Work out the finished part from the listing and answer in its coordinate system (mm). A direction names the side the tool comes from. Coordinates: 2 decimals unless noted, no trailing zeros. Order: outer loops, then holes, each group sorted by start corner. A loop starts at its lowest first (then second) coordinate and runs counter-clockwise, first axis right, second up. Notation, with made-up numbers: M 13.25,14.5 L 66.25,14.5 A28 ccw 66.25,51.5 Z; hole C -23.5,52.25 d3. An arc over 180 degrees is marked long. Use a Markdown table: item, result. Add a question column.
from build123d import *

# Parameters (mm, degrees)
F0_W      = 8
F0_H      = 25
F1_DEPTH  = 1
F2_R      = 6.5
F2_R_2    = 4.3
F3_DEPTH  = 11
F4_R      = 4
F5_R      = 1.35
F6_DEPTH  = 50.001
F7_R      = 2
F8_W      = 1.5
F8_H      = 6
F9_DEPTH  = 2
F11_DEPTH = 2


with BuildPart() as f1:
    # F0 (on Top) → F1 (new body)
    with BuildSketch(Plane.XY):
        with Locations((-4, -12.5)):
            Rectangle(F0_W, F0_H)
        Polygon((-8, 0), (0, 0), (0, 13), (-8, 13), (-42, 13), (-50, 13), (-50, 0), (-42, 0), align=None)
        with Locations((-4, 25.5)):
            Rectangle(F0_W, F0_H)
        with Locations((-46, -12.5)):
            Rectangle(F0_W, F0_H)
        with Locations((-46, 25.5)):
            Rectangle(F0_W, F0_H)
    extrude(amount=F1_DEPTH)

    # F2 (on face) → F3 (join)
    with BuildSketch(Plane.XY.offset(1)):
        with Locations((-34.25, 6.5)):
            Circle(F2_R)
        with Locations((-34.25, 6.5)):
            Circle(F2_R_2, mode=Mode.SUBTRACT)
        with Locations((-15.75, 6.5)):
            Circle(F2_R)
        with Locations((-15.75, 6.5)):
            Circle(F2_R_2, mode=Mode.SUBTRACT)
    extrude(amount=F3_DEPTH)

    # F4
    f4_edges = [f1.edges().sort_by_distance(p)[0] for p in [
        (-38.55, 6.5, 1),
        (-20.05, 6.5, 1),
    ]]
    fillet(f4_edges, radius=F4_R)

    # F5 (on face) → F6 (cut, through all)
    with BuildSketch(Plane.YZ):
        with Locations((6.5, 8.15)):
            Circle(F5_R)
    extrude(amount=-F6_DEPTH, mode=Mode.SUBTRACT)

    # F7
    f7_edges = [f1.edges().sort_by_distance(p)[0] for p in [
        (-42, 38, 0.5),
        (0, 38, 0.5),
        (-8, 38, 0.5),
        (-42, 13, 0.5),
        (-8, 13, 0.5),
        (-8, 0, 0.5),
        (0, -25, 0.5),
        (-8, -25, 0.5),
        (-42, 0, 0.5),
        (-42, -25, 0.5),
        (-50, -25, 0.5),
        (-50, 38, 0.5),
    ]]
    fillet(f7_edges, radius=F7_R)

    # F8 (on face) → F9 (join)
    with BuildSketch(Plane.XY.offset(1)):
        with Locations((-49.25, 33)):
            Rectangle(F8_W, F8_H)
        with Locations((-42.75, 33)):
            Rectangle(F8_W, F8_H)
        with Locations((-42.75, -20)):
            Rectangle(F8_W, F8_H)
        with Locations((-49.25, -20)):
            Rectangle(F8_W, F8_H)
        with Locations((-0.75, 33)):
            Rectangle(F8_W, F8_H)
        with Locations((-7.25, 33)):
            Rectangle(F8_W, F8_H)
        with Locations((-7.25, -20)):
            Rectangle(F8_W, F8_H)
        with Locations((-0.75, -20)):
            Rectangle(F8_W, F8_H)
    extrude(amount=F9_DEPTH)

    # F10 (on face) → F11 (join)
    with BuildSketch(Plane.XY.offset(1)):
        with BuildLine():
            Line((-15.75, 13), (-34.25, 13))
            ThreePointArc((-34.25, 13), (-27.75, 6.5), (-34.25, 0))
            Line((-34.25, 0), (-15.75, 0))
            ThreePointArc((-15.75, 0), (-22.25, 6.5), (-15.75, 13))
        make_face()
    extrude(amount=F11_DEPTH)


solid = f1.part
(1) A cutting plane is placed at A-A on z = 6. Write down the section's boundary in (x, y), plus the area to 3 significant figures.
(2) Which of the six approach directions +Z, -Z, +X, -X, +Y, -Y give full straight-line access (tool end or side, diameter ignored) to faces 1 (the flat face through (-42, -15, 0.8)), 2 (the flat face through (-43, 30, 2)), 3 (the flat face through (-43.5, -20, 2))?
(3) Straight lines are drawn through the part: line 1 (Y direction, x = -16, z = 7.25); line 2 (Z direction, x = -5, y = -6.5); line 3 (Z direction, x = -28.35, y = 6.5). For each, find the intervals that lie inside material, in ascending order.
(4) A cutting plane is placed at C-C on y = 21. Write down the section's boundary in (x, z), plus the area to 3 significant figures.
(5) A cutting plane is placed at D-D on x = -5. Write down the section's boundary in (y, z), plus the area to 3 significant figures.
(6) Given P1, Ø1.2, axis at x = -49.5, y = 33, coming from the +Z side; P2, Ø1.2, axis at x = -7, z = 2, coming from the +Y side; P3, Ø0.8, axis at x = -0.5, z = 1.5, coming from the -Y side; P4, Ø1.5, axis at y = 15, z = 6.5, coming from the -X side, each flat-ended and moving along its own axis, determine where each tip first touches the part or whether it passes through.
(7) The mould has two halves that part along Y. Classify faces 4 (the flat face through (-25, 7, 3)), 5 (the cylindrical face through (-30.28, 4.85, 8.45)), 6 (the cylindrical face through (-42.57, -24.4, 0.51)): pulls with the +Y half, pulls with the -Y half, needs draft (parallel to the pull), parting line crosses it, or undercut.
(8) A cutting plane is placed at B-B on y = -19.5. Write down the section's boundary in (x, z).
From the geometry:
| question | item | result |
|---|---|---|
| 1 | outline | C -34.25,6.5 d13; C -15.75,6.5 d13; hole C -34.25,6.5 d8.6; hole C -15.75,6.5 d8.6 |
| 1 | area | 149 mm2 |
| 2 | face 1 | +Z, -Z, -Y |
| 2 | face 2 | +Z, +X, -X |
| 2 | face 3 | +Z, +Y, -Y |
| 3 | line 1 | y = 0 to 2.21, 10.79 to 13 |
| 3 | line 2 | z = 0 to 1 |
| 3 | line 3 | z = 0 to 6.8, 9.5 to 12 |
| 4 | outline | M -50,0 L -42,0 L -42,1 L -50,1 Z; M -8,0 L 0,0 L 0,1 L -8,1 Z |
| 4 | area | 16.0 mm2 |
| 5 | outline | M -25,0 L 38,0 L 38,1 L -25,1 Z |
| 5 | area | 63.0 mm2 |
| 6 | P1 | stops at z = 3 |
| 6 | P2 | stops at y = 36 |
| 6 | P3 | stops at y = -23 |
| 6 | P4 | passes through |
| 7 | face 4 | needs draft |
| 7 | face 5 | undercut |
| 7 | face 6 | pulls with the -Y half |
| 8 | outline | M -50,0 L -42,0 L -42,3 L -43.5,3 L -43.5,1 L -48.5,1 L -48.5,3 L -50,3 Z; M -8,0 L 0,0 L 0,3 L -1.5,3 L -1.5,1 L -6.5,1 L -6.5,3 L -8,3 Z |
